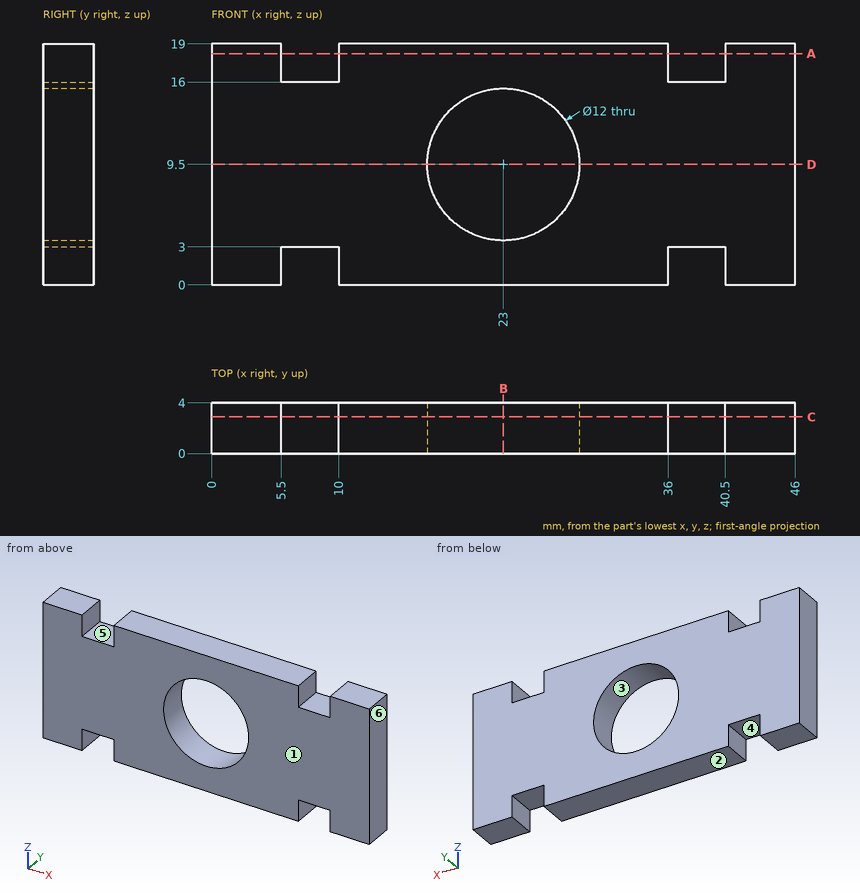
Check sheet for the drawn part. Datum: minimum x, y, z corner. Units: mm. A direction names the side the tool comes from. Coordinates: 2 decimals unless noted, no trailing zeros. Order: outer loops, then holes, each group sorted by start corner. A loop starts at its lowest first (then second) coordinate and runs counter-clockwise, first axis right, second up. Notation, with made-up numbers: (-4.5, 64.5) -> (8.5, 64.5) arc R29 ccw to (8.5, 87.5) -> close; hole circle Ø11 at (-29.5, 11.5). An arc over 180 degrees is marked (long way). Use a Markdown table: item, result. Add a question column.
1. Go/stop test with flat-tipped pins: pin 1 Ø1.5 at (y, z) = (3, 2.5) entering from -X; pin 2 Ø2 at (x, y) = (39, 1.5) entering from +Z; pin 3 Ø9.5 at (x, z) = (23, 9.5) entering from +Y; pin 4 Ø2 at (x, y) = (38.5, 2.5) entering from -Z. Record where each tip stops, or that it passes through.
2. Cross-section at C-C (y = 2.9). Enter the section's corners in (x, z).
3. Material ranges on L1, parallel to X at y = 2.65, z = 18; L2, parallel to X at y = 3.15, z = 9.5; L3, parallel to Z at x = 22, y = 1.25, recorded low to high.
4. Mould release check, pull along Z, two halves, no side actions. Record for the marked faces 1, 2 and 3: pulls with the +Z half, pulls with the -Z half, needs draft (parallel to the pull), parting line crosses it, or undercut.
5. Cross-section at A-A (z = 18.25). Enter the section's corners in (x, y), and give its area (3 significant figures).
6. Cross-section at D-D (z = 9.5). Enter the section's corners in (x, y).
7. Cross-section at B-B (x = 23). Enter the section's corners in (y, z).
8. Set-up check for the marked faces 4, 5 and 6: record each of +Z, -Z, +X, -X, +Y, -Y from which the full face is reachable in a straight line by a thin tool's end or side.
Filled sheet:
| question | item | result |
|---|---|---|
| 1 | pin 1 | x = 0 |
| 1 | pin 2 | z = 16 |
| 1 | pin 3 | through |
| 1 | pin 4 | z = 3 |
| 2 | outline | (0, 0) -> (5.5, 0) -> (5.5, 3) -> (10, 3) -> (10, 0) -> (36, 0) -> (36, 3) -> (40.5, 3) -> (40.5, 0) -> (46, 0) -> (46, 19) -> (40.5, 19) -> (40.5, 16) -> (36, 16) -> (36, 19) -> (10, 19) -> (10, 16) -> (5.5, 16) -> (5.5, 19) -> (0, 19) -> close; hole circle Ø12 at (23, 9.5) |
| 3 | L1 | 0 to 5.5, 10 to 36, 40.5 to 46 |
| 3 | L2 | 0 to 17, 29 to 46 |
| 3 | L3 | 0 to 3.58, 15.42 to 19 |
| 4 | face 1 | needs draft |
| 4 | face 2 | pulls with the -Z half |
| 4 | face 3 | undercut |
| 5 | outline | (0, 0) -> (5.5, 0) -> (5.5, 4) -> (0, 4) -> close; (10, 0) -> (36, 0) -> (36, 4) -> (10, 4) -> close; (40.5, 0) -> (46, 0) -> (46, 4) -> (40.5, 4) -> close |
| 5 | area | 148 mm2 |
| 6 | outline | (0, 0) -> (17, 0) -> (17, 4) -> (0, 4) -> close; (29, 0) -> (46, 0) -> (46, 4) -> (29, 4) -> close |
| 7 | outline | (0, 0) -> (4, 0) -> (4, 3.5) -> (0, 3.5) -> close; (0, 15.5) -> (4, 15.5) -> (4, 19) -> (0, 19) -> close |
| 8 | face 4 | -Z, +Y, -Y |
| 8 | face 5 | +Z, +Y, -Y |
| 8 | face 6 | +Z, -Z, +X, +Y, -Y |
